```python
from build123d import *

# Parameters (mm, degrees)
F0_W     = 310
F0_H     = 180
F1_DEPTH = 15
F2_R     = 3
F3_DEPTH = 15.001


with BuildPart() as f1:
    # F0 (on Right) → F1 (new body)
    with BuildSketch(Plane.YZ):
        with Locations((155, 90)):
            Rectangle(F0_W, F0_H)
    extrude(amount=F1_DEPTH)

    # F2 (on face) → F3 (cut, through all)
    with BuildSketch(Plane.YZ.offset(15)):
        with Locations((7.5, 30)):
            Circle(F2_R)
        with Locations((7.5, 150)):
            Circle(F2_R)
        with Locations((302.5, 150)):
            Circle(F2_R)
        with Locations((302.5, 30)):
            Circle(F2_R)
        with Locations((65, 6)):
            Circle(F2_R)
        with Locations((165, 6)):
            Circle(F2_R)
        with Locations((265, 6)):
            Circle(F2_R)
    extrude(amount=-F3_DEPTH, mode=Mode.SUBTRACT)


solid = f1.part
```
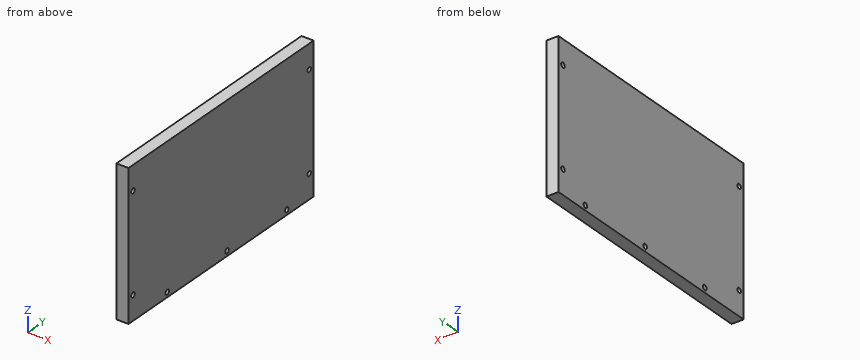
Input: part model. Units: mm. Frame: model coordinates. Give positions to 0.01 mm unless a question says otherwise; leave off trailing zeros. Order: outer loops, then holes, each group sorted by start corner. A loop starts at its lowest first (then second) coordinate and runs counter-clockwise, first axis right, second up. Notation, with made-up numbers: M 45,59 L 52,59 A5 ccw 52,66 Z; hole C 43,58.25 d8. An arc over 180 degrees is marked long. Return JSON: item names as keys, results as strings.
1) Line query: L1, parallel to Y at x = 8, z = 149.5; L2, parallel to Z at x = 3.5, y = 165; L3, parallel to Z at x = 11.5, y = 302.5. Output: solid intervals per line, ascending. Write a range as [from, to].
Taken from the geometry:
{"L1": "y = [0, 4.54], [10.46, 299.54], [305.46, 310]", "L2": "z = [0, 3], [9, 180]", "L3": "z = [0, 27], [33, 147], [153, 180]"}
2) Section query B-B on z = 150. Output: boundary loops of the cut face in (x, y).
Taken from the geometry:
{"outline": "M 0,0 L 15,0 L 15,4.5 L 0,4.5 Z; M 0,10.5 L 15,10.5 L 15,299.5 L 0,299.5 Z; M 0,305.5 L 15,305.5 L 15,310 L 0,310 Z"}
3) Section query C-C on y = 265. Output: boundary loops of the cut face in (x, z).
Taken from the geometry:
{"outline": "M 0,0 L 15,0 L 15,3 L 0,3 Z; M 0,9 L 15,9 L 15,180 L 0,180 Z"}
4) Section query A-A on y = 7.5. Output: boundary loops of the cut face in (x, z), and give its area (3 significant figures).
Taken from the geometry:
{"outline": "M 0,0 L 15,0 L 15,27 L 0,27 Z; M 0,33 L 15,33 L 15,147 L 0,147 Z; M 0,153 L 15,153 L 15,180 L 0,180 Z", "area": "2,520 mm2"}
